from build123d import *

# Parameters (mm, degrees)
BOSS_EXTRUDE1_DEPTH = 4
SKETCH2_R           = 2
SKETCH2_R_2         = 1.5
CUT_EXTRUDE1_DEPTH  = 95.026591983
SKETCH4_W           = 20
SKETCH4_H           = 100
BOSS_EXTRUDE2_DEPTH = 4
FILLET3_R           = 42
FILLET4_R           = 12
SKETCH7_R           = 2
CUT_EXTRUDE3_DEPTH  = 105.120122935
CHAMFER1_SIZE       = 10
FILLET8_R           = 2
CUT_EXTRUDE4_DEPTH  = 105.120122935
CUT_EXTRUDE5_DEPTH  = 105.120122935
SKETCH10_W          = 4
SKETCH10_H          = 35
CUT_EXTRUDE6_DEPTH  = 105.120122935
FILLET9_R           = 3


with BuildPart() as part:
    # Sketch1 → Boss-Extrude1 (new body)
    with BuildSketch(Plane.XY):
        Polygon((-40, 60), (-25, 60), (-25, 52), (-15, 52), (-15, 0), (-21, 0), (-21, -50), (21, -50), (21, 0), (15, 0), (15, 52), (25, 52), (25, 60), (40, 60), (40, -60), (22, -60), (22, -85), (12, -85), (12, -60), (-12, -60), (-12, -85), (-22, -85), (-22, -60), (-40, -60), align=None)
    extrude(amount=BOSS_EXTRUDE1_DEPTH)

    # Sketch2 → Cut-Extrude1 (cut, through all)
    with BuildSketch(Plane(origin=(0, 0, 0), x_dir=(-1, 0, 0), z_dir=(0, 0, -1))):
        with Locations((-28.5, -32)):
            Circle(SKETCH2_R)
        with Locations((17, -56.5)):
            Circle(SKETCH2_R_2)
        with Locations((28.8, -32)):
            Circle(SKETCH2_R)
        with Locations((-17, -56.5)):
            Circle(SKETCH2_R_2)
    extrude(amount=-CUT_EXTRUDE1_DEPTH, mode=Mode.SUBTRACT)

    # Sketch4 → Boss-Extrude2 (add)
    with BuildSketch(Plane.XY.offset(4)):
        with Locations((-50, 10)):
            Rectangle(SKETCH4_W, SKETCH4_H)
        with Locations((50, 10)):
            Rectangle(SKETCH4_W, SKETCH4_H)
    extrude(amount=-BOSS_EXTRUDE2_DEPTH)

    # Fillet3
    # the kernel refuses this fillet: 42 mm, written as the material it takes off along each edge
    with BuildSketch(Plane(origin=(60, 60, 107.531396204), x_dir=(0, -1, 0), z_dir=(0, 0, -1))) as fillet3_piece_1:
        with BuildLine():
            CenterArc((41.412558482, 42), FILLET3_R, 189.594068227, 80.405931773)
            Line((0, 35), (-0.82825117, 34.86))
            ThreePointArc((-0.82825117, 34.86), (-0.84, 17.5), (-0.84, 0))
            Line((-0.84, 0), (0, -0.84))
            Line((0, -0.84), (41.412558482, -0.84))
            Line((41.412558482, -0.84), (41.412558482, 0))
        make_face()
    extrude(amount=211.062792409, mode=Mode.SUBTRACT)
    with BuildSketch(Plane(origin=(-60, 60, 107.531396204), x_dir=(1, 0, 0), z_dir=(0, 0, -1))) as fillet3_piece_2:
        with BuildLine():
            CenterArc((42, 41.412558482), FILLET3_R, 180, 80.405931773)
            Line((0, 41.412558482), (-0.84, 41.412558482))
            Line((-0.84, 41.412558482), (-0.84, 0))
            Line((-0.84, 0), (0, -0.84))
            ThreePointArc((0, -0.84), (17.5, -0.84), (34.86, -0.82825117))
            Line((34.86, -0.82825117), (35, 0))
        make_face()
    extrude(amount=211.062792409, mode=Mode.SUBTRACT)

    # Fillet4
    fillet4_edges = [part.edges().sort_by_distance(p)[0] for p in [
        (60, -40, 2),
        (-60, -40, 2),
    ]]
    fillet(fillet4_edges, radius=FILLET4_R)

    # Sketch7 → Cut-Extrude3 (cut, through all)
    with BuildSketch(Plane.XY):
        with Locations(Location((-55, -20, 0), (0, 0, 180))):
            Circle(SKETCH7_R)
        with Locations(Location((55, -20, 0), (0, 0, 180))):
            Circle(SKETCH7_R)
        with Locations(Location((-37, -20, 0), (0, 0, 180))):
            Circle(SKETCH7_R)
        with Locations(Location((37, -20, 0), (0, 0, 180))):
            Circle(SKETCH7_R)
    extrude(amount=CUT_EXTRUDE3_DEPTH, mode=Mode.SUBTRACT)

    # Chamfer1
    chamfer1_edges = [part.edges().sort_by_distance(p)[0] for p in [
        (-40, -60, 2),
        (40, -60, 2),
    ]]
    chamfer(chamfer1_edges, length=CHAMFER1_SIZE)

    # Fillet8
    fillet8_edges = [part.edges().sort_by_distance(p)[0] for p in [
        (-30, -60, 2),
        (-40, -50, 2),
        (30, -60, 2),
        (40, -50, 2),
        (40, -40, 2),
        (-40, -40, 2),
    ]]
    fillet(fillet8_edges, radius=FILLET8_R)

    # Sketch8 → Cut-Extrude4 (cut, through all)
    with BuildSketch(Plane(origin=(0, 0, 0), x_dir=(-1, 0, 0), z_dir=(0, 0, -1))):
        with BuildLine():
            ThreePointArc((-17.964817996, 17.438774634), (-30.770630407, 21.535466224), (-44.214817996, 21.375674028))
            ThreePointArc((-44.214817996, 21.375674028), (-45.841525426, 19.061841075), (-43.527692473, 17.435133644))
            ThreePointArc((-43.527692473, 17.435133644), (-31.363903701, 17.579707536), (-19.777692473, 13.87317705))
            ThreePointArc((-19.777692473, 13.87317705), (-17.088456442, 14.749538603), (-17.964817996, 17.438774634))
        make_face()
        with BuildLine():
            ThreePointArc((17.964817996, 17.438774634), (30.770630407, 21.535466224), (44.214817996, 21.375674028))
            ThreePointArc((44.214817996, 21.375674028), (45.841525426, 19.061841075), (43.527692473, 17.435133644))
            ThreePointArc((43.527692473, 17.435133644), (31.363903701, 17.579707536), (19.777692473, 13.87317705))
            ThreePointArc((19.777692473, 13.87317705), (17.088456442, 14.749538603), (17.964817996, 17.438774634))
        make_face()
    extrude(amount=-CUT_EXTRUDE4_DEPTH, mode=Mode.SUBTRACT)

    # Sketch9 → Cut-Extrude5 (cut, through all)
    with BuildSketch(Plane.XY.offset(4)):
        Polygon((-24, 52), (-20, 52), (-20, 45.2), (-18.25, 45.2), (-18.25, 42), (-25.75, 42), (-25.75, 45.2), (-24, 45.2), align=None)
    cut_extrude5 = extrude(amount=-CUT_EXTRUDE5_DEPTH, mode=Mode.SUBTRACT)

    # Mirror1: Cut-Extrude5 across plane
    add(cut_extrude5.mirror(Plane(origin=(0, 0, 0), x_dir=(0, 0, 1), z_dir=(1, 0, 0))), mode=Mode.SUBTRACT)

    # Sketch10 → Cut-Extrude6 (cut, through all)
    with BuildSketch(Plane.XY.offset(4)):
        with Locations((46, -22.5)):
            Rectangle(SKETCH10_W, SKETCH10_H)
        Polygon((49.827462353, 0.296846572), (49.827462353, -3.703153428), (56.485281374, -3.703153428), (54.371414492, 20.296846572), (50.355929074, 20.296846572), (52.117484809, 0.296846572), align=None)
    cut_extrude6 = extrude(amount=-CUT_EXTRUDE6_DEPTH, mode=Mode.SUBTRACT)

    # Mirror2: Cut-Extrude6 across plane
    add(cut_extrude6.mirror(Plane(origin=(0, 0, 0), x_dir=(0, 0, 1), z_dir=(1, 0, 0))), mode=Mode.SUBTRACT)

    # Fillet9
    # the kernel refuses this fillet: 3 mm, written as the material it adds along each edge
    with BuildSketch(Plane(origin=(56.485281374, -3.703153428, 4), x_dir=(-1, 0, 0), z_dir=(0, 0, -1))) as fillet9_piece_1:
        with BuildLine():
            CenterArc((FILLET9_R * 1.09194914132, FILLET9_R), FILLET9_R, 174.966503844, 95.033496156)
            Line((FILLET9_R * 0.0958055662996, FILLET9_R * 1.08773812138), (0, 0))
            Line((0, 0), (FILLET9_R * 1.09194914132, 0))
        make_face()
    extrude(amount=4)
    with BuildSketch(Plane(origin=(-56.485281374, -3.703153428, 4), x_dir=(1, 0, 0), z_dir=(0, 0, -1))) as fillet9_piece_2:
        with BuildLine():
            CenterArc((FILLET9_R * 1.09194914132, -FILLET9_R), FILLET9_R, 90, 95.033496156)
            Line((FILLET9_R * 0.0958055662996, -FILLET9_R * 1.08773812138), (0, 0))
            Line((0, 0), (FILLET9_R * 1.09194914132, 0))
        make_face()
    extrude(amount=4)
    # the kernel refuses this fillet: 3 mm, written as the material it takes off along each edge
    with BuildSketch(Plane(origin=(52.117484809, 0.296846572, 11.783837895), x_dir=(-1, 0, 0), z_dir=(0, 0, -1))) as fillet9_2_piece_1:
        with BuildLine():
            CenterArc((3.261606451, 2.838313679), FILLET9_R, 174.966503844, 76.136892771)
            Line((0.273175726, 3.101528043), (0, 0))
            Line((0, 0), (2.290022456, 0))
        make_face()
    extrude(amount=19.56767579, mode=Mode.SUBTRACT)
    with BuildSketch(Plane(origin=(48, -40, 14.146118724), x_dir=(0, 1, 0), z_dir=(0, 0, -1))) as fillet9_2_piece_2:
        with BuildLine():
            CenterArc((3.514718626, 3), FILLET9_R, 160.528779366, 109.471220634)
            ThreePointArc((0.686291501, 4), (0.172817284, 2.029223745), (0, 0))
            Line((0, 0), (3.514718626, 0))
        make_face()
    extrude(amount=24.292237447, mode=Mode.SUBTRACT)
    with BuildSketch(Plane(origin=(44, -40, 11.247448714), x_dir=(-0.9998582920116396, -0.01683436650328442, 0), z_dir=(0, 0, -1))) as fillet9_2_piece_3:
        with BuildLine():
            CenterArc((2.950772393, 2.949071777), FILLET9_R, 180.964583715, 78.463040967)
            Line((-0.048802483, 2.898568677), (-0.348759971, 2.893518367))
            Line((-0.348759971, 2.893518367), (-0.299957488, -0.00505031))
            Line((-0.299957488, -0.00505031), (0.00505031, -0.299957488))
            ThreePointArc((0.00505031, -0.299957488), (2.004766894, -0.266288755), (2.345296923, -0.294907178))
            Line((2.345296923, -0.294907178), (2.400340147, 0))
        make_face()
    extrude(amount=18.494897428, mode=Mode.SUBTRACT)
    with BuildSketch(Plane(origin=(-44, -40, 11.247448714), x_dir=(0, 1, 0), z_dir=(0, 0, -1))) as fillet9_2_piece_4:
        with BuildLine():
            CenterArc((2.898979486, 3), FILLET9_R, 191.536959033, 78.463040967)
            Line((-0.040408206, 2.4), (-0.334346975, 2.34))
            ThreePointArc((-0.334346975, 2.34), (-0.3, 2), (-0.3, 0))
            Line((-0.3, 0), (0, -0.3))
            Line((0, -0.3), (2.898979486, -0.3))
            Line((2.898979486, -0.3), (2.898979486, 0))
        make_face()
    extrude(amount=18.494897428, mode=Mode.SUBTRACT)
    with BuildSketch(Plane(origin=(-48, -40, 14.146118724), x_dir=(-0.9855985596534866, 0.16910197872577487, 0), z_dir=(0, 0, -1))) as fillet9_2_piece_5:
        with BuildLine():
            CenterArc((3.551141553, 2.956795679), FILLET9_R, 170.264389683, 109.471220634)
            Line((0.594345874, 3.464101615), (0, 0))
            ThreePointArc((0, 0), (2.029223745, -0.172817284), (4.058447489, 0))
        make_face()
    extrude(amount=24.292237447, mode=Mode.SUBTRACT)
    with BuildSketch(Plane(origin=(-52.117484809, 0.296846572, 11.783837895), x_dir=(0.08773812137778342, 0.9961435750217422, 0), z_dir=(0, 0, -1))) as fillet9_2_piece_6:
        with BuildLine():
            CenterArc((3.113535158, 3), FILLET9_R, 193.863107229, 76.136892771)
            Line((0.200922268, 2.281191156), (0, 0))
            Line((0, 0), (3.113535158, 0))
        make_face()
    extrude(amount=19.56767579, mode=Mode.SUBTRACT)


solid = part.part
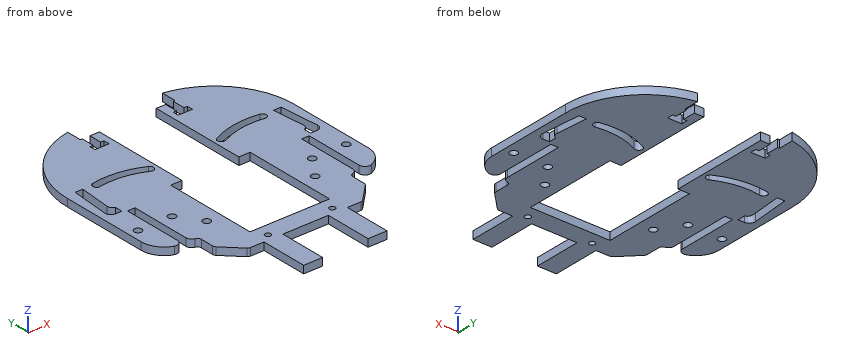
Input: part model. Units: mm. Frame: model coordinates. Coordinates: 2 decimals unless noted, no trailing zeros. Order: outer loops, then holes, each group sorted by start corner. A loop starts at its lowest first (then second) coordinate and runs counter-clockwise, first axis right, second up. Notation, with made-up numbers: M -38.5,32.25 L 15.5,32.25 A35 cw 15.5,71.25 Z; hole C 63.5,33 d1. An arc over 180 degrees is marked long. Write item = value, one per line. Start each with the question number.
(1) First-contact query: P1, Ø1.2, axis at y = 22, z = 1, coming from the +X side; P2, Ø1.2, axis at x = -51.5, z = 2, coming from the -Y side. Flat tips, straight axial feed; report the tip coordinate or a pass-through.
(2) Section A-A on y = -75.5. Output: boundary loops of the cut face in (x, z).
(3) Section C-C on x = -37. Output: boundary loops of the cut face in (y, z), and give its area (3 significant figures).
(4) Section B-B on y = -20. Give the number of separate pieces and of enclosed holes in the cut face, and give its area (3 significant figures).
(5) Line query: line 1 along X through (y, z) = (-11.5, 2.3); line 2 along X through (y, z) = (-79, 3.8); line 3 along X through (y, z) = (-57, 1.8). Output: solid intervals per line, ascending. Write a range as [from, to].
(6) Section D-D on y = 10.5. Output: boundary loops of the cut face in (x, z).
Result set:
q1.P1 = 59.91
q1.P2 = -39.49
q2.outline = M -22,0 L -12,0 L -12,4 L -22,4 Z; M 12,0 L 22,0 L 22,4 L 12,4 Z
q3.outline = M -53,0 L -22,0 L -22,4 L -53,4 Z; M -18,0 L 18,0 L 18,4 L -18,4 Z; M 22,0 L 56.04,0 L 56.04,4 L 22,4 Z
q3.area = 404 mm²
q4.separate_pieces = 8
q4.enclosed_holes = 0
q4.area = 216 mm²
q5.line_1 = [-60, -48], [-44, -21], [21, 44], [48, 60]
q5.line_2 = [-22, -12], [12, 22]
q5.line_3 = [-33, -18.41], [-15.59, 15.59], [18.41, 33]
q6.outline = M -60,0 L -55.23,0 L -55.23,4 L -60,4 Z; M -51.22,0 L -15,0 L -15,4 L -51.22,4 Z; M 15,0 L 51.22,0 L 51.22,4 L 15,4 Z; M 55.23,0 L 60,0 L 60,4 L 55.23,4 Z
